Read the model definition and answer for the solid it produces. Units are mm, in the model's axes. A direction names the side the tool comes from. Coordinates: 2 decimals unless noted, no trailing zeros. Order: outer loops, then holes, each group sorted by start corner. A loop starts at its lowest first (then second) coordinate and runs counter-clockwise, first axis right, second up. Notation, with made-up numbers: (-1.5, -34) - (8.5, -34) arc R15 cw to (8.5, -11) - close; hole circle Ø10 at (67, 47). An arc over 180 degrees is marked (long way). Use one line per item in the form item = value.
```python
from build123d import *

# Parameters (mm, degrees)
SKETCH1_W              = 304.8
SKETCH1_H              = 152.4
SKETCH1_R              = 3.175
BOARD_DEPTH            = 2.54
SKETCH2_W              = 66.548
SKETCH2_H              = 102.87
ACCELNET_DEPTH         = 24.892
SKETCH3_W              = 53.086
SKETCH3_H              = 11.43
D25TOCOMPUTER_DEPTH    = 12.7
SKETCH5_W              = 39.116
SKETCH5_H              = 11.43
D15TOMOTOR_BRAKE_DEPTH = 12.7
SKETCH7_W              = 19.05
SKETCH7_H              = 8.89
SKETCH7_R              = 2.286
SKETCH7_W_2            = 30.175587071
SKETCH7_H_2            = 6.35
SKETCH7_R_2            = 1.524
HVIN_24VIN_5VIN_DEPTH  = 6.35
SKETCH9_W              = 8.89
SKETCH9_H              = 45.72
SKETCH9_R              = 2.286
MOTORS_BRAKES_DEPTH    = 6.35
SKETCH10_W             = 12.7
SKETCH10_H             = 152.4
SKETCH10_R             = 3.175
PLATEDEDGE_DEPTH       = 0.0254


with BuildPart() as part:
    # Sketch1 → Board (new body)
    with BuildSketch(Plane(origin=(0, 0, 0), x_dir=(1, 0, 0), z_dir=(0, 1, 0))):
        with Locations((152.4, 76.2)):
            Rectangle(SKETCH1_W, SKETCH1_H)
        with Locations(Location((298.731278283, 76.2, 0), (0, 0, 270))):
            Circle(SKETCH1_R, mode=Mode.SUBTRACT)
        with Locations(Location((298.731278283, 133.35, 0), (0, 0, 270))):
            Circle(SKETCH1_R, mode=Mode.SUBTRACT)
        with Locations(Location((298.731278283, 19.05, 0), (0, 0, 90))):
            Circle(SKETCH1_R, mode=Mode.SUBTRACT)
        with Locations(Location((6.068721717, 19.05, 0), (0, 0, 270))):
            Circle(SKETCH1_R, mode=Mode.SUBTRACT)
        with Locations(Location((6.068721717, 76.2, 0), (0, 0, 90))):
            Circle(SKETCH1_R, mode=Mode.SUBTRACT)
        with Locations(Location((6.068721717, 133.35, 0), (0, 0, 90))):
            Circle(SKETCH1_R, mode=Mode.SUBTRACT)
    extrude(amount=BOARD_DEPTH)

    # Sketch2 → Accelnet (add)
    with BuildSketch(Plane(origin=(0, 2.54, 0), x_dir=(-1, 0, 0), z_dir=(0, 1, 0))):
        with Locations((-63.093174763, -79.48542652)):
            Rectangle(SKETCH2_W, SKETCH2_H)
        with Locations((-151.798661476, -79.48542652)):
            Rectangle(SKETCH2_W, SKETCH2_H)
    extrude(amount=ACCELNET_DEPTH)

    # Sketch3 → D25toComputer (add)
    with BuildSketch(Plane(origin=(0, 2.54, 0), x_dir=(-1, 0, 0), z_dir=(0, 1, 0))):
        with Locations((-75.767610713, -144.145)):
            Rectangle(SKETCH3_W, SKETCH3_H)
    extrude(amount=D25TOCOMPUTER_DEPTH)

    # Sketch5 → D15toMotor/Brake (add)
    with BuildSketch(Plane(origin=(0, 2.54, 0), x_dir=(-1, 0, 0), z_dir=(0, 1, 0))):
        with Locations((-177.038519959, -144.145)):
            Rectangle(SKETCH5_W, SKETCH5_H)
        with Locations((-223.715302991, -144.145)):
            Rectangle(SKETCH5_W, SKETCH5_H)
    extrude(amount=D15TOMOTOR_BRAKE_DEPTH)

    # Sketch7 → HVin/24Vin/5Vin (add)
    # profile 1 of 2: a face of its own
    with BuildSketch(Plane(origin=(0, 2.54, 0), x_dir=(-1, 0, 0), z_dir=(0, 1, 0))):
        with Locations((-263.099763315, -29.684886318)):
            Rectangle(SKETCH7_W, SKETCH7_H)
        with Locations(Location((-258.354389381, -29.684886318, 0), (0, 0, 90))):
            Circle(SKETCH7_R, mode=Mode.SUBTRACT)
        with Locations(Location((-267.845137249, -29.684886318, 0), (0, 0, 270))):
            Circle(SKETCH7_R, mode=Mode.SUBTRACT)
    # profile 2 of 2: a face of its own
    with BuildSketch(Plane(origin=(0, 2.54, 0), x_dir=(-1, 0, 0), z_dir=(0, 1, 0))):
        with Locations((-263.099763315, -44.067178792)):
            Rectangle(SKETCH7_W_2, SKETCH7_H_2)
        with Locations(Location((-266.938051441, -44.067178792, 0), (0, 0, 90))):
            Circle(SKETCH7_R_2, mode=Mode.SUBTRACT)
        with Locations(Location((-274.531114606, -44.067178792, 0), (0, 0, 270))):
            Circle(SKETCH7_R_2, mode=Mode.SUBTRACT)
        with Locations(Location((-251.668412024, -44.067178792, 0), (0, 0, 90))):
            Circle(SKETCH7_R_2, mode=Mode.SUBTRACT)
        with Locations(Location((-259.261475189, -44.067178792, 0), (0, 0, 270))):
            Circle(SKETCH7_R_2, mode=Mode.SUBTRACT)
    extrude(amount=HVIN_24VIN_5VIN_DEPTH)

    # Sketch9 → Motors/Brakes (add)
    # profile 1 of 2: a face of its own
    with BuildSketch(Plane(origin=(0, 2.54, 0), x_dir=(-1, 0, 0), z_dir=(0, 1, 0))):
        with Locations((-272.10570634, -86.062744457)):
            Rectangle(SKETCH9_W, SKETCH9_H)
        with Locations(Location((-272.10570634, -73.524162022, 0), (0, 0, 90))):
            Circle(SKETCH9_R, mode=Mode.SUBTRACT)
        with Locations(Location((-272.10570634, -67.174162022, 0), (0, 0, 90))):
            Circle(SKETCH9_R, mode=Mode.SUBTRACT)
        with Locations(Location((-272.10570634, -86.224162022, 0), (0, 0, 90))):
            Circle(SKETCH9_R, mode=Mode.SUBTRACT)
        with Locations(Location((-272.10570634, -79.874162022, 0), (0, 0, 90))):
            Circle(SKETCH9_R, mode=Mode.SUBTRACT)
        with Locations(Location((-272.10570634, -98.924162022, 0), (0, 0, 90))):
            Circle(SKETCH9_R, mode=Mode.SUBTRACT)
        with Locations(Location((-272.10570634, -92.574162022, 0), (0, 0, 90))):
            Circle(SKETCH9_R, mode=Mode.SUBTRACT)
        with Locations(Location((-272.10570634, -105.274162022, 0), (0, 0, 90))):
            Circle(SKETCH9_R, mode=Mode.SUBTRACT)
    # profile 2 of 2: a face of its own
    with BuildSketch(Plane(origin=(0, 2.54, 0), x_dir=(-1, 0, 0), z_dir=(0, 1, 0))):
        with Locations((-253.05570634, -86.062744457)):
            Rectangle(SKETCH9_W, SKETCH9_H)
        with Locations(Location((-253.05570634, -79.874162022, 0), (0, 0, 90))):
            Circle(SKETCH9_R, mode=Mode.SUBTRACT)
        with Locations(Location((-253.05570634, -67.174162022, 0), (0, 0, 90))):
            Circle(SKETCH9_R, mode=Mode.SUBTRACT)
        with Locations(Location((-253.05570634, -98.924162022, 0), (0, 0, 90))):
            Circle(SKETCH9_R, mode=Mode.SUBTRACT)
        with Locations(Location((-253.05570634, -105.274162022, 0), (0, 0, 90))):
            Circle(SKETCH9_R, mode=Mode.SUBTRACT)
        with Locations(Location((-253.05570634, -73.524162022, 0), (0, 0, 90))):
            Circle(SKETCH9_R, mode=Mode.SUBTRACT)
        with Locations(Location((-253.05570634, -86.224162022, 0), (0, 0, 90))):
            Circle(SKETCH9_R, mode=Mode.SUBTRACT)
        with Locations(Location((-253.05570634, -92.574162022, 0), (0, 0, 90))):
            Circle(SKETCH9_R, mode=Mode.SUBTRACT)
    extrude(amount=MOTORS_BRAKES_DEPTH)

    # Sketch10 → platedEdge (add)
    # profile 1 of 2: a face of its own
    with BuildSketch(Plane(origin=(0, 2.54, 0), x_dir=(-1, 0, 0), z_dir=(0, 1, 0))):
        with Locations((-298.45, -76.2)):
            Rectangle(SKETCH10_W, SKETCH10_H)
        with Locations(Location((-298.731278283, -133.35, 0), (0, 0, 90))):
            Circle(SKETCH10_R, mode=Mode.SUBTRACT)
        with Locations(Location((-298.731278283, -76.2, 0), (0, 0, 90))):
            Circle(SKETCH10_R, mode=Mode.SUBTRACT)
        with Locations(Location((-298.731278283, -19.05, 0), (0, 0, 270))):
            Circle(SKETCH10_R, mode=Mode.SUBTRACT)
    # profile 2 of 2: a face of its own
    with BuildSketch(Plane(origin=(0, 2.54, 0), x_dir=(-1, 0, 0), z_dir=(0, 1, 0))):
        with Locations((-6.35, -76.2)):
            Rectangle(SKETCH10_W, SKETCH10_H)
        with Locations(Location((-6.068721717, -19.05, 0), (0, 0, 90))):
            Circle(SKETCH10_R, mode=Mode.SUBTRACT)
        with Locations(Location((-6.068721717, -76.2, 0), (0, 0, 270))):
            Circle(SKETCH10_R, mode=Mode.SUBTRACT)
        with Locations(Location((-6.068721717, -133.35, 0), (0, 0, 270))):
            Circle(SKETCH10_R, mode=Mode.SUBTRACT)
    extrude(amount=PLATEDEDGE_DEPTH)


solid = part.part
```
(1) Section D-D, the plane x = 176 is taken. Write down the section's boundary in (y, z).
Answer list:
outline = (0, -152.4) - (2.54, -152.4) - (2.54, -149.86) - (15.24, -149.86) - (15.24, -138.43) - (2.54, -138.43) - (2.54, -130.92) - (27.43, -130.92) - (27.43, -28.05) - (2.54, -28.05) - (2.54, 0) - (0, 0) - close
(2) Straight lines are drawn through the part: L1, parallel to X at y = 14, z = -97; L2, parallel to Z at x = 35.5, y = 17.75; L3, parallel to Z at x = 65.5, y = 4. For each, find the intervals that lie inside material, in ascending order.
Answer list:
L1 = 29.82 to 96.37, 118.52 to 185.07
L2 = -130.92 to -28.05
L3 = -149.86 to -138.43, -130.92 to -28.05
(3) Section A-A, the plane z = -19.05 is taken. State how many separate pieces and enclosed holes the cut face has, then the cut area to 3 significant figures.
Answer list:
separate_pieces = 3
enclosed_holes = 0
area = 742 mm2
(4) Given pin 1 Ø3 at (x, z) = (153.5, -52.5) entering from -Y; pin 2 Ø3.5 at (y, z) = (9.5, -147) entering from +X; pin 3 Ø5.5 at (x, z) = (180.5, -145) entering from +Y; pin 4 Ø6 at (x, z) = (127, -21.5) entering from +Y, each flat-ended and moving along its own axis, determine where each tip first touches the part or whether it passes through.
Answer list:
pin_1 = 0
pin_2 = 243.27
pin_3 = 15.24
pin_4 = 2.54
(5) Which of the six approach directions +Z, -Z, +X, -X, +Y, -Y give full straight-line access (tool end or side, diameter ignored) to faces 5 (the flat face through (267.661, 6, -86)), 6 (the flat face through (256, 8.89, -86)), 7 (the flat face through (224, 9, -138.43)), 8 (the flat face through (248.012, 6, -44))?
Answer list:
face_5 = -Z, +Y
face_6 = +Z, -Z, +X, +Y
face_7 = +Z, +X, -X, +Y
face_8 = +Z, -Z, +Y
(6) Section B-B, the plane y = 24.5 is taken. Write down the section's boundary in (x, z).
Answer list:
outline = (29.82, -130.92) - (96.37, -130.92) - (96.37, -28.05) - (29.82, -28.05) - close; (118.52, -130.92) - (185.07, -130.92) - (185.07, -28.05) - (118.52, -28.05) - close
(7) The mould has two halves that part along Z. Classify faces 1 (the flat face through (185.073, 15, -80)), 2 (the flat face through (263, 6, -25.24)), 3 (the flat face through (272, 6, -63.203)), 4 (the flat face through (253, 6, -63.203)): +Z half, -Z half, draft (parallel to the pull), parting line (faces both ways), or undercut.
Answer list:
face_1 = draft
face_2 = +Z half
face_3 = undercut
face_4 = undercut
